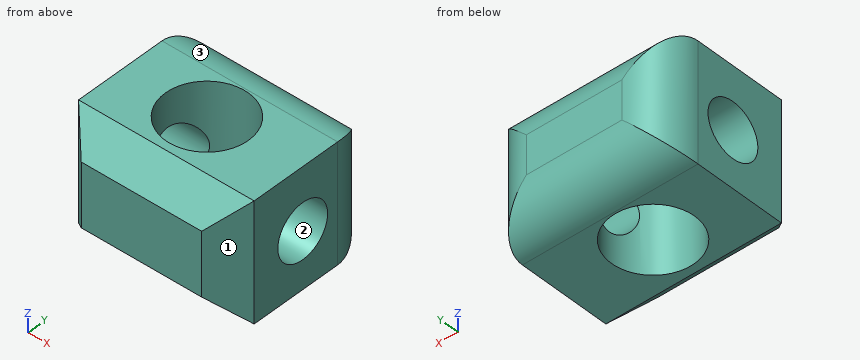
from build123d import *

# Parameters (mm, degrees)
F1_W     = 63.614873
F1_H     = 42.992467
F2_DEPTH = 58
F3_R     = 14.485281
F4_SIZE  = 10
F6_D     = 30
F8_D     = 20


with BuildPart() as f2:
    # F1 (on face) → F2 (new body)
    with BuildSketch(Plane.XZ):
        with Locations((4.01963, 1.048599)):
            Rectangle(F1_W, F1_H)
    extrude(amount=-F2_DEPTH)

    # F3
    f3_edges = [f2.edges().sort_by_distance(p)[0] for p in [
        (-27.787806, 58, 1.048599),
        (4.01963, 58, 22.544833),
        (35.827067, 58, 1.048599),
        (4.01963, 58, -20.447634),
    ]]
    fillet(f3_edges, radius=F3_R)

    # F4
    f4_edges = [f2.edges().sort_by_distance(p)[0] for p in [
        (35.827067, 0, 1.048599),
        (4.01963, 0, -20.447634),
        (-27.787806, 0, 1.048599),
        (4.01963, 0, 22.544833),
    ]]
    chamfer(f4_edges, length=F4_SIZE)

    # F6 (through all)
    with Locations(Plane.XY.offset(22.544833)):
        with Locations((2.594914, 27.867122)):
            Hole(F6_D / 2)

    # F8 (through all)
    with Locations(Plane(origin=(-27.787806, 0, 0), x_dir=(0, -1, 0), z_dir=(-1, 0, 0))):
        with Locations((-29.496336, 0)):
            Hole(F8_D / 2)


solid = f2.part
Verification items for the finished model (mm, model axes). Face numbers are marked on the shaded views. Give positions to 0.01 mm unless a question says otherwise; leave off trailing zeros. Loops run counter-clockwise (first coordinate to the right, second up) from the corner with the lowest first, then second, coordinate; pieces in that order, holes last.
1) Thickness scan on line 1 along X through (y, z) = (40.5, 19.5); line 2 along Y through (x, z) = (5.5, -6); line 3 along Z through (x, y) = (-23.5, 27.5). Record the ranges inside material, lowest first.
2) Sectioned sample at B-B, the plane x = -10. Enter the section's corners in (y, z), then the cut area to 3 significant figures.
3) Sectioned sample at A-A, the plane y = 21. Enter the section's corners in (x, z).
4) Sectioned sample at D-D, the plane x = 31.5. Enter the section's corners in (y, z), then the cut area to 3 significant figures.
5) Draft check along Y on the marked faces 1, 2 and 3. Enter one of: pulls with the +Y half, pulls with the -Y half, needs draft (parallel to the pull), parting line crosses it, or undercut.
6) Sectioned sample at C-C, the plane z = 5. Enter the section's corners in (x, y).
7) Depth check by flat-ended pin: pin 1 Ø4 at (x, z) = (-5.5, 17) entering from +Y; pin 2 Ø18 at (y, z) = (29.5, 0) entering from -X; pin 3 Ø1.5 at (y, z) = (48.5, -11) entering from -X; pin 4 Ø8 at (x, y) = (-1.5, 14.5) entering from -Z. Enter the tip coordinate at first touch or a pass-through.
Answers:
1. line 1: x = -27.79 to -5.49, 10.68 to 35.83
1. line 2: y = 0 to 13.15, 42.58 to 58
1. line 3: z = -20.45 to -9.8, 9.8 to 22.54
2. outline: (0, -10.45) - (10, -20.45) - (19.72, -20.45) - (19.72, -2.11) arc R10 cw to (19.72, 2.11) - (19.72, 22.54) - (10, 22.54) - (0, 12.54) - close; (36.01, -20.45) - (43.51, -20.45) arc R14.49 ccw to (58, -5.96) - (58, 8.06) arc R14.49 ccw to (43.51, 22.54) - (36.01, 22.54) - (36.01, 7.58) arc R10 cw to (36.01, -7.58) - close
2. area: 1,570 mm2
3. outline: (-27.79, -20.45) - (-10.74, -20.45) - (-10.74, -5.27) - (-27.79, -5.27) - close; (-27.79, 5.27) - (-10.74, 5.27) - (-10.74, 22.54) - (-27.79, 22.54) - close; (15.93, -20.45) - (35.83, -20.45) - (35.83, -5.27) - (15.93, -5.27) - close; (15.93, 5.27) - (35.83, 5.27) - (35.83, 22.54) - (15.93, 22.54) - close
4. outline: (5.67, -16.12) - (10, -20.45) - (43.51, -20.45) arc R14.49 ccw to (53.84, -16.12) - (53.84, 18.22) arc R14.49 ccw to (43.51, 22.54) - (10, 22.54) - (5.67, 18.22) - close; hole circle Ø20 at (29.5, 0)
4. area: 1,710 mm2
5. face 1: pulls with the -Y half
5. face 2: undercut
5. face 3: pulls with the +Y half
6. outline: (-27.79, 10) - (-17.79, 0) - (25.83, 0) - (35.83, 10) - (35.83, 20.84) - (15.84, 20.84) arc R15 cw to (-10.66, 20.84) - (-27.79, 20.84) - close; (-27.79, 38.16) - (-8.32, 38.16) arc R15 cw to (13.51, 38.16) - (35.83, 38.16) - (35.83, 43.51) arc R14.49 ccw to (21.34, 58) - (-13.3, 58) arc R14.49 ccw to (-27.79, 43.51) - close
7. pin 1: stops at y = 56.23
7. pin 2: passes through
7. pin 3: stops at x = -27.15
7. pin 4: stops at z = -20.45
